```python
from build123d import *

# Parameters (mm, degrees)
SKETCH1_R                  = 4.7625
BOSS_EXTRUDE1_DEPTH        = 17.018
SKETCH2_R                  = 3.175
BOSS_EXTRUDE2_DEPTH        = 6.35
SKETCH4_R                  = 2.413
BOSS_EXTRUDE3_DEPTH        = 7.112
SKETCH5_R                  = 3.19405
CUT_EXTRUDE2_DEPTH         = 5.842
CHAMFER1_SIZE              = 0.254
FILLET1_R                  = 0.254
CHAMFER2_SIZE              = 0.508
F_10_24_TAPPED_HOLE1_D     = 3.7973
F_10_24_TAPPED_HOLE1_DEPTH = 8.89
F_10_24_TAPPED_HOLE1_TIP   = 1.140824014
CHAMFER3_SIZE              = 0.508
SKETCH10_W                 = 0.762
SKETCH10_H                 = 1.5875
FILLET2_R                  = 0.254


with BuildPart() as part:
    # Sketch1 → Boss-Extrude1 (new body)
    with BuildSketch(Plane.XY):
        Circle(SKETCH1_R)
    extrude(amount=BOSS_EXTRUDE1_DEPTH)

    # Sketch2 → Boss-Extrude2 (add)
    with BuildSketch(Plane.XY.offset(17.018)):
        Circle(SKETCH2_R)
    extrude(amount=BOSS_EXTRUDE2_DEPTH)

    # Sketch4 → Boss-Extrude3 (add)
    with BuildSketch(Plane.XY.offset(23.368)):
        Circle(SKETCH4_R)
    extrude(amount=BOSS_EXTRUDE3_DEPTH)

    # Sketch5 → Cut-Extrude2 (cut)
    with BuildSketch(Plane(origin=(0, 0, 0), x_dir=(-1, 0, 0), z_dir=(0, 0, -1))):
        Circle(SKETCH5_R)
    extrude(amount=-CUT_EXTRUDE2_DEPTH, mode=Mode.SUBTRACT)

    # Chamfer1
    chamfer1_edges = [part.edges().sort_by_distance(p)[0] for p in [
        (3.19405, 0, 0),
    ]]
    chamfer(chamfer1_edges, length=CHAMFER1_SIZE)

    # Fillet1
    fillet1_edges = [part.edges().sort_by_distance(p)[0] for p in [
        (3.19405, 0, 5.842),
    ]]
    fillet(fillet1_edges, radius=FILLET1_R)

    # Chamfer2
    chamfer2_edges = [part.edges().sort_by_distance(p)[0] for p in [
        (-3.175, 0, 23.368),
    ]]
    chamfer(chamfer2_edges, length=CHAMFER2_SIZE)

    # #10-24 Tapped Hole1
    with Locations(Plane(origin=(0, 0, 5.842), x_dir=(-1, 0, 0), z_dir=(0, 0, -1))):
        with Locations((0, 0)):
            Hole(F_10_24_TAPPED_HOLE1_D / 2, depth=F_10_24_TAPPED_HOLE1_DEPTH)
            with Locations((0, 0, -(F_10_24_TAPPED_HOLE1_DEPTH + F_10_24_TAPPED_HOLE1_TIP / 2))):  # 118° drill point
                Cone(0, F_10_24_TAPPED_HOLE1_D / 2, F_10_24_TAPPED_HOLE1_TIP, mode=Mode.SUBTRACT)

    # Chamfer3
    chamfer3_edges = [part.edges().sort_by_distance(p)[0] for p in [
        (-2.413, 0, 30.48),
    ]]
    chamfer(chamfer3_edges, length=CHAMFER3_SIZE)

    # Sketch10 → Cut-Revolve1 (revolve, cut)
    with BuildSketch(Plane(origin=(0, 0, 0), x_dir=(1, 0, 0), z_dir=(0, 1, 0))):
        with Locations((-2.032, -24.16175)):
            Rectangle(SKETCH10_W, SKETCH10_H)
    revolve(axis=Axis((0, 0, 29.927585912), (0, 0, -1)), mode=Mode.SUBTRACT)

    # Fillet2
    fillet2_edges = [part.edges().sort_by_distance(p)[0] for p in [
        (-3.175, 0, 17.018),
    ]]
    fillet(fillet2_edges, radius=FILLET2_R)


solid = part.part
```
Verification items for the finished model (mm, model axes). A direction names the side the tool comes from. Give positions to 0.01 mm unless a question says otherwise; leave off trailing zeros. Loops run counter-clockwise (first coordinate to the right, second up) from the corner with the lowest first, then second, coordinate; pieces in that order, holes last. Notation, with made-up numbers: M -8.75,72 L 25.25,72 A19 ccw 25.25,81 Z; hole C 7.5,-36 d6. An arc over 180 degrees is marked long. Return JSON: item names as keys, results as strings.
1) Gauge pin test, flat ends, axial feed: P1, Ø5, axis at x = 0.5, z = 26.5, coming from the +Y side; P2, Ø2, axis at y = 3.5, z = 19, coming from the -X side; P3, Ø1, axis at y = 3.5, z = 9.5, coming from the +X side. Record the tip position at first contact, or that the pin passes through.
Findings:
{"P1": "stops at y = 2.41", "P2": "stops at x = -1.96", "P3": "stops at x = 3.7"}
2) Mould release check, pull along Y, two halves, no side actions. Record for faces 6 (the flat face through (-1, -2, 24.956)), 7 (the cylindrical face through (-3.047, 0.959, 2.884)), 8 (the cylindrical face through (-0.69, -3.1, 20.03)): released by +Y, released by -Y, zero draft, split by the parting line, or undercut.
Findings:
{"face 6": "zero draft", "face 7": "undercut", "face 8": "split by the parting line"}
3) Tool access check on faces 1 (the flat face through (2, 3, 0)), 2 (the flat face through (-2, -1, 5.842)), 3 (the cylindrical face through (-3.78, -2.9, 8.39)), 4 (the cylindrical face through (-1.525, -0.632, 24.151)), 5 (the cylindrical face through (-1.915, -1.468, 27.429)). Record the directions out of +Z, -Z, +X, -X, +Y, -Y that give a thin tool (end or side, any length) a straight path to the whole face; none if there is none.
Findings:
{"face 1": "-Z, +X, -X, +Y, -Y", "face 2": "-Z", "face 3": "+Z, -Z", "face 4": "none", "face 5": "+Z"}
4) Material ranges on L1, parallel to Y at x = 0, z = 11.5; L2, parallel to Y at x = 0, z = 2.25; L3, parallel to Z at x = 3, y = 1.75, recorded low to high. Write a range as [from, to].
Findings:
{"L1": "y = [-4.76, -1.9], [1.9, 4.76]", "L2": "y = [-4.76, -3.19], [3.19, 4.76]", "L3": "z = [0, 17.02]"}
5) Section check A-A, the plane z = 10.5. Enter the section's corners in (x, y) (1 decimal), and give its area (3 significant figures).
Findings:
{"outline": "C 0,0 d9.5; hole C 0,0 d3.8", "area": "59.9 mm2"}
6) Section check C-C, the plane z = 15. Enter the section's corners in (x, y) (1 decimal).
Findings:
{"outline": "C 0,0 d9.5; hole C 0,0 d2.9"}
7) Section check B-B, the plane z = 22. Enter the section's corners in (x, y) (3 decimals).
Findings:
{"outline": "C 0,0 d6.35"}
